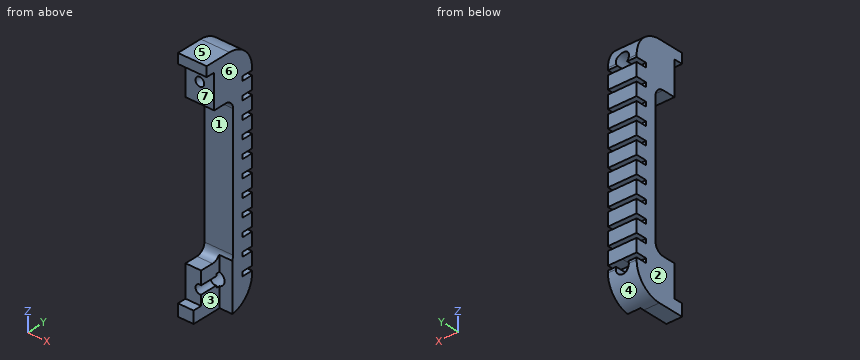
```python
from build123d import *

# Parameters (mm, degrees)
SKETCH_1_W          = 6.6
SKETCH_1_H          = 54
SKETCH_1_R          = 1.49999954
EXTRUDE_1_DEPTH     = 12
FILLET_1_R          = 6
SKETCH_2_W          = 34
SKETCH_2_H          = 14
CUT_EXTRUDE_1_DEPTH = 20
FILLET_2_R          = 2
SKETCH_3_W          = 1
SKETCH_3_H          = 2.5
CUT_EXTRUDE_2_DEPTH = 31.274742098
SKETCH_4_W          = 14.557801868
SKETCH_4_H          = 49
CUT_EXTRUDE_3_DEPTH = 2
SKETCH_6_R          = 1.5
SKETCH_6_R_2        = 1
SKETCH_6_R_3        = 1.49999954
EXTRUDE_2_DEPTH     = 4
SKETCH_7_W          = 6
SKETCH_7_H          = 22
CUT_EXTRUDE_4_DEPTH = 6.8


with BuildPart() as part:
    # 草图1 → 凸台-拉伸1 (new body)
    with BuildSketch(Plane(origin=(0, 0, 0), x_dir=(1, 0, 0), z_dir=(0, 1, 0))):
        with Locations((-25, 0)):
            Rectangle(SKETCH_1_W, SKETCH_1_H)
        with Locations(Location((-25, -21.49999992, 0), (0, 0, 270))):
            Circle(SKETCH_1_R, mode=Mode.SUBTRACT)
        with Locations(Location((-25, 20.9999989, 0), (0, 0, 270))):
            Circle(SKETCH_1_R, mode=Mode.SUBTRACT)
    extrude(amount=EXTRUDE_1_DEPTH)

    # 圆角1
    # the kernel refuses this fillet: 6 mm, written as the material it takes off along each edge
    with BuildSketch(Plane(origin=(-6.7, 12, 27), x_dir=(0, -1, 0), z_dir=(-1, 0, 0)), Plane(origin=(-43.3, 12, -27), x_dir=(0, -1, 0), z_dir=(1, 0, 0))) as fillet_1_piece_1:
        with BuildLine():
            CenterArc((FILLET_1_R, -FILLET_1_R), FILLET_1_R, 90, 90)
            Line((0, -FILLET_1_R), (0, 0))
            Line((0, 0), (FILLET_1_R, 0))
        make_face()
    extrude(amount=36.6, mode=Mode.SUBTRACT)

    # 草图2 → 切除-拉伸1 (cut)
    with BuildSketch(Plane.ZY.offset(28.3)):
        Rectangle(SKETCH_2_W, SKETCH_2_H)
    extrude(amount=-CUT_EXTRUDE_1_DEPTH, mode=Mode.SUBTRACT)

    # 圆角2
    fillet_2_edges = [part.edges().sort_by_distance(p)[0] for p in [
        (-25, 7, 17),
        (-25, 7, -17),
    ]]
    fillet(fillet_2_edges, radius=FILLET_2_R)

    # 草图3 → 切除-拉伸2 (cut, through all)
    with BuildSketch(Plane.ZY.offset(28.3)):
        with Locations((0, 10.75)):
            Rectangle(SKETCH_3_W, SKETCH_3_H)
        with Locations((4, 10.75)):
            Rectangle(SKETCH_3_W, SKETCH_3_H)
        with Locations((8, 10.75)):
            Rectangle(SKETCH_3_W, SKETCH_3_H)
        with Locations((12, 10.75)):
            Rectangle(SKETCH_3_W, SKETCH_3_H)
        with Locations((16, 10.75)):
            Rectangle(SKETCH_3_W, SKETCH_3_H)
        with Locations((20, 10.75)):
            Rectangle(SKETCH_3_W, SKETCH_3_H)
        with Locations((-4, 10.75)):
            Rectangle(SKETCH_3_W, SKETCH_3_H)
        with Locations((-8, 10.75)):
            Rectangle(SKETCH_3_W, SKETCH_3_H)
        with Locations((-12, 10.75)):
            Rectangle(SKETCH_3_W, SKETCH_3_H)
        with Locations((-16, 10.75)):
            Rectangle(SKETCH_3_W, SKETCH_3_H)
        with Locations((-20, 10.75)):
            Rectangle(SKETCH_3_W, SKETCH_3_H)
    extrude(amount=-CUT_EXTRUDE_2_DEPTH, mode=Mode.SUBTRACT)

    # 草图4 → 切除-拉伸3 (cut)
    with BuildSketch(Plane.XZ):
        with Locations((-25, 0.25000051)):
            Rectangle(SKETCH_4_W, SKETCH_4_H)
    extrude(amount=-CUT_EXTRUDE_3_DEPTH, mode=Mode.SUBTRACT)

    # 草图6 → 凸台-拉伸2 (add)
    # profile 1 of 2: a face of its own
    with BuildSketch(Plane.XZ.offset(-2)):
        with Locations(Location((-25, 21.49999992, 0), (0, 0, 270))):
            Circle(SKETCH_6_R)
        with Locations(Location((-25, 21.49999992, 0), (0, 0, 270))):
            Circle(SKETCH_6_R_2, mode=Mode.SUBTRACT)
    # profile 2 of 2: a face of its own
    with BuildSketch(Plane.XZ.offset(-2)):
        with Locations(Location((-25, -20.9999989, 0), (0, 0, 270))):
            Circle(SKETCH_6_R_3)
        with Locations(Location((-25, -20.9999989, 0), (0, 0, 270))):
            Circle(SKETCH_6_R_2, mode=Mode.SUBTRACT)
    extrude(amount=-EXTRUDE_2_DEPTH)

    # 草图7 → 切除-拉伸4 (cut)
    with BuildSketch(Plane.XZ):
        with Locations((-21.7, -27)):
            Rectangle(SKETCH_7_W, SKETCH_7_H)
    extrude(amount=-CUT_EXTRUDE_4_DEPTH, mode=Mode.SUBTRACT)


solid = part.part
```
Part model, mm, in its own coordinate system. Face numbers are marked on the shaded views. A direction names the side the tool comes from. Round coordinates to 2 decimals unless told otherwise and drop trailing zeros. Order: outer loops, then holes, each group sorted by start corner. A loop starts at its lowest first (then second) coordinate and runs counter-clockwise, first axis right, second up. Notation, with made-up numbers: M 84,35 L 96,35 A17 ccw 96,62 Z; hole C 33.5,52.25 d4. An arc over 180 degrees is marked long. Answer in a Markdown table with one row per item. Add a question column.
Q1. Mould opens along Z. For the marked faces 4, 5, 6 and 7 say: +Z half, -Z half, draft (parallel to the pull), parting line (faces both ways), or undercut.
Q2. Pin check, flat tips, straight feed: pin 1 (3 mm diameter, centred on x = -24, y = 10, fed in from +Z); pin 2 (2 mm diameter, centred on x = -25, y = 10, fed in from -Z); pin 3 (2 mm diameter, centred on x = -25, y = 8, fed in from -Z); pin 4 (4 mm diameter, centred on y = 3.5, z = 11.5, fed in from -X). Stop position of each tip, or through.
Q3. Cut at B-B on z = 21.5. Give the cut face in (x, y).
Q4. 3-axis set-ups, long thin cutter, end or side, ignore diameter. For the marked faces 1, 2 and 3: which of +Z, -Z, +X, -X, +Y, -Y reach the whole face in a straight line?
Q5. Cut at C-C on z = 7. Give the cut face in (x, y).
Q6. Wall check: L1, parallel to Z at x = -25, y = 8.25; L2, parallel to Z at x = -25, y = 7.75; L3, parallel to Y at x = -25, z = -9. Give the ranges that are in metal, low to high. Write a range as from..to.
Q7. Cut at D-D on y = 8. Give the cut face in (x, z).
Q8. Cut at A-A on y = 4.25. Give the cut face in (x, z).
Established:
| question | item | result |
|---|---|---|
| 1 | face 4 | -Z half |
| 1 | face 5 | +Z half |
| 1 | face 6 | draft |
| 1 | face 7 | undercut |
| 2 | pin 1 | stops at z = 26.45 |
| 2 | pin 2 | stops at z = -26.2 |
| 2 | pin 3 | stops at z = -26.92 |
| 2 | pin 4 | passes through |
| 3 | outline | M -28.3,2 L -26,2 L -26,6 L -26.5,6 L -26.5,11.98 L -28.3,11.98 Z; M -24,2 L -21.7,2 L -21.7,11.98 L -23.5,11.98 L -23.5,6 L -24,6 Z |
| 4 | face 1 | +X, -X, -Y |
| 4 | face 2 | +Z, -Z, -X, +Y, -Y |
| 4 | face 3 | -Z, +X, -Y |
| 5 | outline | M -28.3,7 L -21.7,7 L -21.7,12 L -28.3,12 Z |
| 6 | L1 | z = -26.56..-22.5, -19.5..20, 23..26.56 |
| 6 | L2 | z = -26.74..-22.5, -19.5..20, 23..26.74 |
| 6 | L3 | y = 7..12 |
| 7 | outline | M -28.3,-26.66 L -21.7,-26.66 L -21.7,26.66 L -28.3,26.66 Z; hole C -25,-21 d3; hole C -25,21.5 d3 |
| 8 | outline | M -28.3,-27 L -24.7,-27 L -24.7,-21.95 A1 cw long -24.7,-20.05 L -24.7,-17 L -28.3,-17 Z; M -28.3,17 L -21.7,17 L -21.7,27 L -28.3,27 Z; hole C -25,21.5 d2 |
